```python
from build123d import *

# Parameters (mm, degrees)
BOSS_EXTRUDE1_DEPTH = 12.7
SKETCH2_R           = 4.7625
BOSS_EXTRUDE2_DEPTH = 7.62
SKETCH3_R           = 6.35
BOSS_EXTRUDE3_DEPTH = 33.528
SKETCH8_R           = 6.35
CUT_EXTRUDE3_DEPTH  = 12.319
SKETCH9_R           = 2.667
CUT_EXTRUDE4_DEPTH  = 3.81


with BuildPart() as part:
    # Sketch1 → Boss-Extrude1 (new body)
    with BuildSketch(Plane(origin=(0, 0, 0), x_dir=(1, 0, 0), z_dir=(0, 1, 0))):
        Polygon((6.35, -3.666174209), (6.35, 3.666174209), (0, 7.332348419), (-6.35, 3.666174209), (-6.35, -3.666174209), (0, -7.332348419), align=None)
    extrude(amount=BOSS_EXTRUDE1_DEPTH)

    # Sketch2 → Boss-Extrude2 (add)
    with BuildSketch(Plane.XZ):
        Circle(SKETCH2_R)
    extrude(amount=BOSS_EXTRUDE2_DEPTH)

    # Sketch3 → Boss-Extrude3 (add)
    with BuildSketch(Plane(origin=(0, 12.7, 0), x_dir=(1, 0, 0), z_dir=(0, 1, 0))):
        Circle(SKETCH3_R)
    extrude(amount=BOSS_EXTRUDE3_DEPTH)

    # Sketch6 → Tapped Hole1 (revolve, cut)
    with BuildSketch(Plane(origin=(0, 46.228, 0), x_dir=(0, 0, 1), z_dir=(1, 0, 0))):
        Polygon((0, 0), (0, 20.263317848), (2.0193, 19.05), (2.0193, 16.002), (2.413, 16.002), (2.413, 3.506322905), (5.461, 0), align=None)
    revolve(axis=Axis((0, 52.578, 0), (0, -1, 0)), mode=Mode.SUBTRACT)

    # Sketch8 → Cut-Extrude3 (cut)
    with BuildSketch(Plane(origin=(0, 46.228, 0), x_dir=(1, 0, 0), z_dir=(0, 1, 0))):
        Circle(SKETCH8_R)
        Polygon((-4.7625, -2.749630657), (0, -5.499261314), (4.7625, -2.749630657), (4.7625, 2.749630657), (0, 5.499261314), (-4.7625, 2.749630657), align=None, mode=Mode.SUBTRACT)
    extrude(amount=-CUT_EXTRUDE3_DEPTH, mode=Mode.SUBTRACT)

    # Sketch9 → Cut-Extrude4 (cut)
    with BuildSketch(Plane(origin=(0, 46.228, 0), x_dir=(-1, 0, 0), z_dir=(0, -1, 0))):
        Circle(SKETCH9_R)
    extrude(amount=CUT_EXTRUDE4_DEPTH, mode=Mode.SUBTRACT)


solid = part.part
```
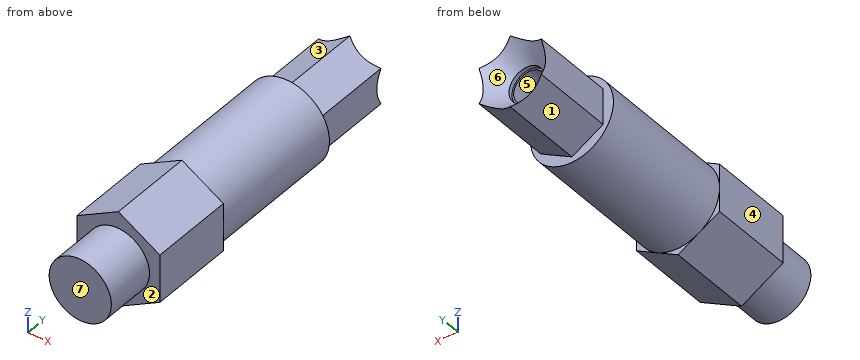
Read the model definition and answer for the solid it produces. Units are mm, in the model's axes. Face numbers are marked on the shaded views. A direction names the side the tool comes from. Coordinates: 2 decimals unless noted, no trailing zeros. Write each loop counter-clockwise with the first axis right and the second up, starting at its lowest first coordinate (ties: lowest second). Pieces come first, ordered by that corner, then holes. Notation, with made-up numbers: (29.5, 83.5) -> (57.5, 83.5) arc R30 cw to (57.5, 105.5) -> close; hole circle Ø10 at (-34, -39.5). An arc over 180 degrees is marked (long way). Write item = value, one per line.
(1) Section B-B on y = 2.5 is taken. Write down the section's boundary in (x, z).
From the geometry:
outline = (-6.35, -3.67) -> (0, -7.33) -> (6.35, -3.67) -> (6.35, 3.67) -> (0, 7.33) -> (-6.35, 3.67) -> close
(2) Given pin 1 Ø5 at (x, z) = (-3, 3) entering from +Y; pin 2 Ø1 at (x, z) = (4, -3) entering from +Y; pin 3 Ø4 at (x, z) = (0.5, 0) entering from +Y; pin 4 Ø6 at (y, z) = (42, 0.5) entering from -X, each flat-ended and moving along its own axis, determine where each tip first touches the part or whether it passes through.
From the geometry:
pin_1 = 46.23
pin_2 = 46.1
pin_3 = 42.42
pin_4 = -4.76
(3) Section A-A on y = 39 is taken. Write down the section's boundary in (x, z), plus the area to 3 significant figures.
From the geometry:
outline = (-4.76, -2.75) -> (0, -5.5) -> (4.76, -2.75) -> (4.76, 2.75) -> (0, 5.5) -> (-4.76, 2.75) -> close; hole circle Ø4.83 at (0, 0)
area = 60.3 mm2
(4) Straight lines are drawn through the part: L1, parallel to X at y = 42.6, z = 0; L2, parallel to Z at x = 0, y = 35.5; L3, parallel to X at y = 28.95, z = 0. For each, find the intervals that lie inside material, in ascending order. Write a range as from..to.
From the geometry:
L1 = -4.76..-2.67, 2.67..4.76
L2 = -5.5..-2.41, 2.41..5.5
L3 = -6.35..-2.02, 2.02..6.35
(5) For a pull along X with two mould halves and no side action, classify the marked faces 4, 5, 6 and 7 as +X half, -X half, draft (parallel to the pull), parting line (faces both ways), or undercut.
From the geometry:
face_4 = -X half
face_5 = undercut
face_6 = undercut
face_7 = draft
(6) Which of the six approach directions +Z, -Z, +X, -X, +Y, -Y give full straight-line access (tool end or side, diameter ignored) to the marked faces 1, 2 and 3?
From the geometry:
face_1 = -Z, -X, +Y
face_2 = -Y
face_3 = +Z, -X, +Y
(7) Section C-C on y = 24.5 is taken. Write down the section's boundary in (x, z), plus the area to 3 significant figures.
From the geometry:
outline = circle Ø12.7 at (0, 0)
area = 127 mm2
